The figure shows three views and two pictorial views of one solid part (mm, origin at its lowest corner). Answer the questions. A direction names the side the tool comes from. Round coordinates to 2 decimals unless told otherwise and drop trailing zeros. Order: outer loops, then holes, each group sorted by start corner. A loop starts at its lowest first (then second) coordinate and runs counter-clockwise, first axis right, second up. Notation, with made-up numbers: (-28.5, 4) -> (23.5, 4) arc R31 cw to (23.5, 37) -> close; hole circle Ø9 at (89, -30.75). An arc over 180 degrees is marked (long way). Answer as a JSON object with one key per item and string values. Group by question number.
Item 1: Given P1, Ø11.5, axis at x = 45, z = 38.5, coming from the -Y side, flat-ended and moving along its own axis, determine where the tip first touches the part or whether it passes through.
Item 2: Section D-D, the plane x = 55.5 is taken. Write down the section's boundary in (y, z).
Item 3: Section B-B, the plane z = 40 is taken. Write down the section's boundary in (x, y), plus the area to 3 significant figures.
Item 4: For the marked faces 1 and 2, determine the directions among +Z, -Z, +X, -X, +Y, -Y from which every point of the face is accessible in a straight line to the end or side of a thin tool.
Item 5: Section A-A, the plane x = 38 is taken. Write down the section's boundary in (y, z).
Item 6: The mould has two halves that part along X. Classify the marked faces 3 and 4: pulls with the +X half, pulls with the -X half, needs draft (parallel to the pull), parting line crosses it, or undercut.
Item 7: Consider probe 1 along Z at (x, y) = (38, 0.95); probe 2 along X at (y, z) = (5.3, 40); probe 3 along Z at (x, y) = (38, 3.2). Determine where each line is inside the solid, lowest interval first. Write a range as from..to.
Item 8: Section C-C, the plane y = 6 is taken. Write down the section's boundary in (x, z).
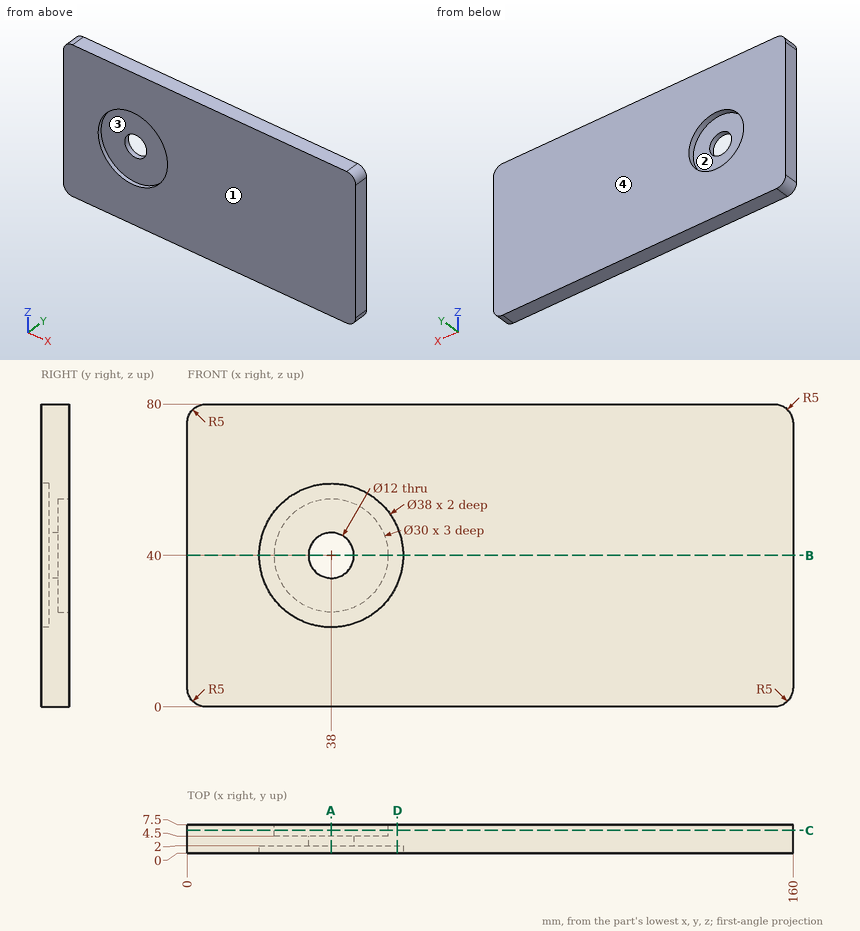
Values found:
{
 "1": {"P1": "y = 2"},
 "2": {"outline": "(0, 0) -> (7.5, 0) -> (7.5, 80) -> (0, 80) -> (0, 47.4) -> (2, 47.4) -> (2, 32.6) -> (0, 32.6) -> close"},
 "3": {"outline": "(0, 0) -> (19, 0) -> (19, 2) -> (32, 2) -> (32, 4.5) -> (23, 4.5) -> (23, 7.5) -> (0, 7.5) -> close; (44, 2) -> (57, 2) -> (57, 0) -> (160, 0) -> (160, 7.5) -> (53, 7.5) -> (53, 4.5) -> (44, 4.5) -> close", "area": "1,000 mm2"},
 "4": {"face 1": "+Z, -Z, +X, -X, -Y", "face 2": "+Y"},
 "5": {"outline": "(0, 0) -> (7.5, 0) -> (7.5, 25) -> (4.5, 25) -> (4.5, 34) -> (2, 34) -> (2, 21) -> (0, 21) -> close; (0, 59) -> (2, 59) -> (2, 46) -> (4.5, 46) -> (4.5, 55) -> (7.5, 55) -> (7.5, 80) -> (0, 80) -> close"},
 "6": {"face 3": "undercut", "face 4": "needs draft"},
 "7": {"probe 1": "0..21, 59..80", "probe 2": "0..23, 53..160", "probe 3": "0..34, 46..80"},
 "8": {"outline": "(0, 5) arc R5 ccw to (5, 0) -> (155, 0) arc R5 ccw to (160, 5) -> (160, 75) arc R5 ccw to (155, 80) -> (5, 80) arc R5 ccw to (0, 75) -> close; hole circle Ø30 at (38, 40)"}
}
